```python
from build123d import *

# Parameters (mm, degrees)
SKETCH1_R           = 11.049
BOSS_EXTRUDE1_DEPTH = 25.4
SKETCH2_R           = 12.7
BOSS_EXTRUDE2_DEPTH = 6.35
SKETCH5_R           = 11.176
CUT_EXTRUDE2_DEPTH  = 5.545328
SKETCH6_R           = 7.27456
CUT_EXTRUDE3_DEPTH  = 0.1999996
SKETCH3_R           = 5.500000049
CUT_EXTRUDE1_DEPTH  = 37.477972806
CHAMFER1_SIZE       = 0.299999908


with BuildPart() as part:
    # Sketch1 → Boss-Extrude1 (new body)
    with BuildSketch(Plane(origin=(0, 0, 0), x_dir=(1, 0, 0), z_dir=(0, 1, 0))):
        with Locations(Location((0, 0, 0), (0, 0, 270))):
            Circle(SKETCH1_R)
    extrude(amount=BOSS_EXTRUDE1_DEPTH)

    # Sketch2 → Boss-Extrude2 (add)
    with BuildSketch(Plane.XZ):
        with Locations(Location((0, 0, 0), (0, 0, 270))):
            Circle(SKETCH2_R)
    extrude(amount=BOSS_EXTRUDE2_DEPTH)

    # Sketch5 → Cut-Extrude2 (cut)
    with BuildSketch(Plane.XZ.offset(6.35)):
        with Locations(Location((0, 0, 0), (0, 0, 270))):
            Circle(SKETCH5_R)
    extrude(amount=-CUT_EXTRUDE2_DEPTH, mode=Mode.SUBTRACT)

    # Sketch6 → Cut-Extrude3 (cut)
    with BuildSketch(Plane.XZ.offset(0.804672)):
        with Locations(Location((0, 0, 0), (0, 0, 270))):
            Circle(SKETCH6_R)
    extrude(amount=-CUT_EXTRUDE3_DEPTH, mode=Mode.SUBTRACT)

    # Sketch3 → Cut-Extrude1 (cut, through all)
    with BuildSketch(Plane.XZ.offset(6.35)):
        with Locations(Location((0, 0, 0), (0, 0, 270))):
            Circle(SKETCH3_R)
    extrude(amount=-CUT_EXTRUDE1_DEPTH, mode=Mode.SUBTRACT)

    # Chamfer1
    chamfer1_edges = [part.edges().sort_by_distance(p)[0] for p in [
        (0, -6.35, 11.176),
        (0, -0.6046724, 5.500000049),
        (0, 25.4, 5.500000049),
        (0, 25.4, -11.049),
        (0, 0, 12.7),
        (0, -6.35, 12.7),
    ]]
    chamfer(chamfer1_edges, length=CHAMFER1_SIZE)


solid = part.part
```
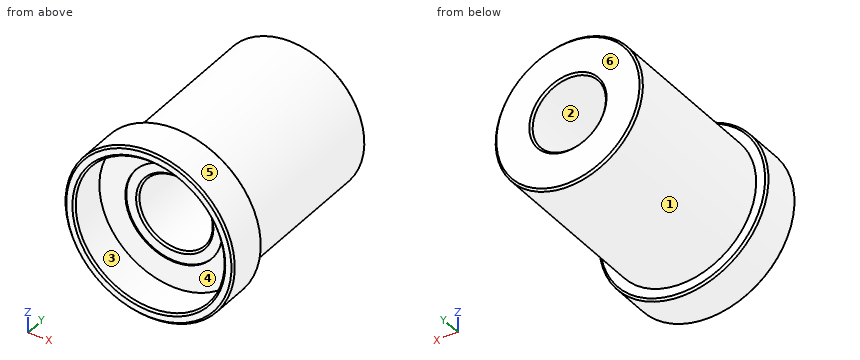
CAD build for the part. Positions are in the model's coordinates, mm. Face numbers are marked on the shaded views. A direction names the side the tool comes from. Round coordinates to 2 decimals unless told otherwise and drop trailing zeros. Order: outer loops, then holes, each group sorted by start corner. A loop starts at its lowest first (then second) coordinate and runs counter-clockwise, first axis right, second up.
Item 1: Probe line 1 along X through (y, z) = (-0.7, 0); line 2 along X through (y, z) = (-3.2, 0); line 3 along Y through (x, z) = (10, -3.25). List the from-to ranges inside material, lowest first.
Item 2: Tool access for the marked faces 1, 2 and 3: list every direction of +Z, -Z, +X, -X, +Y, -Y with a clear straight run to the whole face (end or side of a thin tool).
Item 3: Pin check, flat tips, straight feed: pin 1 (6.5 mm diameter, centred on x = 0, z = 0, fed in from -Y); pin 2 (1 mm diameter, centred on x = -3.5, y = 12, fed in from -Z); pin 3 (1 mm diameter, centred on y = 12.5, z = 6, fed in from +X); pin 4 (1.5 mm diameter, centred on x = -1.5, y = 10, fed in from -Z). Stop position of each tip, or through.
Item 4: Mould opens along Z. For the marked faces 4, 5 and 6 say: pulls with the +Z half, pulls with the -Z half, needs draft (parallel to the pull), parting line crosses it, or undercut.
Item 5: Saw through at C-C on y = 8.5. Write the cut outline in (x, z), then the cut area to 3 significant figures.
Reported:
1. line 1: x = -12.7 to -7.27, 7.27 to 12.7
1. line 2: x = -12.7 to -11.18, 11.18 to 12.7
1. line 3: y = -0.8 to 25.4
2. face 1: +Y
2. face 2: +Y, -Y
2. face 3: -Y
3. pin 1: passes through
3. pin 2: stops at z = -10.63
3. pin 3: stops at x = 9.58
3. pin 4: stops at z = -11.02
4. face 4: undercut
4. face 5: parting line crosses it
4. face 6: needs draft
5. outline: circle Ø22.1 at (0, 0); hole circle Ø11 at (0, 0)
5. area: 288 mm2
